Here's how the part is built. I have some questions about the finished solid (model axes, mm). Face numbers are marked on the shaded views. A direction names the side the tool comes from. Round coordinates to 2 decimals unless told otherwise and drop trailing zeros. Order: outer loops, then holes, each group sorted by start corner. A loop starts at its lowest first (then second) coordinate and runs counter-clockwise, first axis right, second up. Notation, with made-up numbers: (-3, 23.25) -> (56, 23.25) arc R8 cw to (56, 29.25) -> close; hole circle Ø2 at (70, -23). An arc over 180 degrees is marked (long way). Answer in a Markdown table with one row per item.
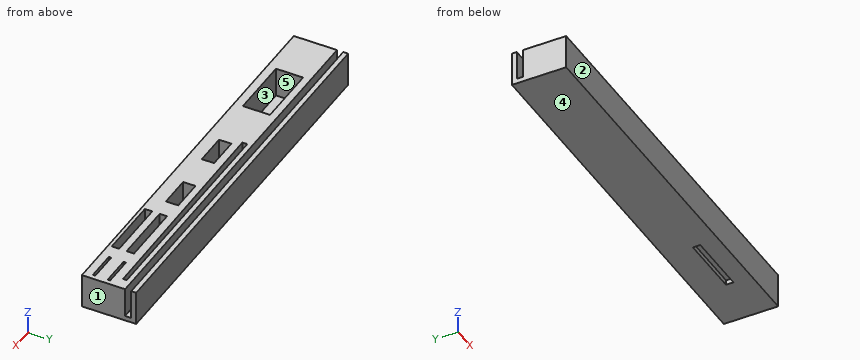
```python
from build123d import *

# Parameters (mm, degrees)
F0_W     = 160
F0_H     = 17.5
F0_W_2   = 25
F0_H_2   = 11
F0_W_3   = 13
F0_H_3   = 5
F0_H_4   = 3
F0_W_4   = 12
F0_H_5   = 1
F0_H_6   = 2.5
F0_H_7   = 2
F1_DEPTH = 2
F2_DEPTH = 12
F3_DEPTH = 2
F4_DEPTH = 2


# Not quite as in the source:
# - a feature names something its author has since deleted; it is built from what else it names


with BuildPart() as f1:
    # F0 (on Top) → F1 (new body)
    with BuildSketch(Plane.XY):
        with Locations((-35.2099549949, 29.3164705649)):
            Rectangle(F0_W, F0_H)
        with Locations((-82.7099549949, 29.5664705649)):
            Rectangle(F0_W_2, F0_H_2, mode=Mode.SUBTRACT)
        with Locations((-42.2099549949, 28.443671599)):
            Rectangle(F0_W_3, F0_H_3, mode=Mode.SUBTRACT)
        with Locations((12.2900450051, 23.443671599)):
            Rectangle(F0_W_2, F0_H_4, mode=Mode.SUBTRACT)
        with Locations((36.7900450051, 24.443671599)):
            Rectangle(F0_W_4, F0_H_5, mode=Mode.SUBTRACT)
        with Locations((-14.2099549949, 28.943671599)):
            Rectangle(F0_W_3, F0_H_3, mode=Mode.SUBTRACT)
        with Locations((12.2900450051, 29.443671599)):
            Rectangle(F0_W_2, F0_H_4, mode=Mode.SUBTRACT)
        with Locations((36.7900450051, 30.443671599)):
            Rectangle(F0_W_4, F0_H_5, mode=Mode.SUBTRACT)
        Polygon((-51.2099549949, 36.0664705649), (39.7900450051, 36.0664705649), (39.7900450051, 34.5664705649), (-51.2099549949, 34.0664705649), align=None, mode=Mode.SUBTRACT)
        with Locations((-35.2099549949, 39.3164705649)):
            Rectangle(F0_W, F0_H_6)
        with Locations((-35.2099549949, 41.5664705649)):
            Rectangle(F0_W, F0_H_7)
        with Locations((-82.7099549949, 29.5664705649)):
            Rectangle(F0_W_2, F0_H_2)
        Polygon((39.7900450051, 34.5664705649), (39.7900450051, 36.0664705649), (-51.2099549949, 36.0664705649), (-51.2099549949, 34.0664705649), align=None)
        with Locations((12.2900450051, 23.443671599)):
            Rectangle(F0_W_2, F0_H_4)
        with Locations((-42.2099549949, 28.443671599)):
            Rectangle(F0_W_3, F0_H_3)
        with Locations((-14.2099549949, 28.943671599)):
            Rectangle(F0_W_3, F0_H_3)
        with Locations((36.7900450051, 24.443671599)):
            Rectangle(F0_W_4, F0_H_5)
        with Locations((36.7900450051, 30.443671599)):
            Rectangle(F0_W_4, F0_H_5)
    extrude(amount=-F1_DEPTH)

    # F0 (on Top) → F2 (join)
    with BuildSketch(Plane.XY):
        with Locations((-35.2099549949, 29.3164705649)):
            Rectangle(F0_W, F0_H)
        with Locations((-82.7099549949, 29.5664705649)):
            Rectangle(F0_W_2, F0_H_2, mode=Mode.SUBTRACT)
        with Locations((-42.2099549949, 28.443671599)):
            Rectangle(F0_W_3, F0_H_3, mode=Mode.SUBTRACT)
        with Locations((12.2900450051, 23.443671599)):
            Rectangle(F0_W_2, F0_H_4, mode=Mode.SUBTRACT)
        with Locations((36.7900450051, 24.443671599)):
            Rectangle(F0_W_4, F0_H_5, mode=Mode.SUBTRACT)
        with Locations((-14.2099549949, 28.943671599)):
            Rectangle(F0_W_3, F0_H_3, mode=Mode.SUBTRACT)
        with Locations((12.2900450051, 29.443671599)):
            Rectangle(F0_W_2, F0_H_4, mode=Mode.SUBTRACT)
        with Locations((36.7900450051, 30.443671599)):
            Rectangle(F0_W_4, F0_H_5, mode=Mode.SUBTRACT)
        Polygon((-51.2099549949, 36.0664705649), (39.7900450051, 36.0664705649), (39.7900450051, 34.5664705649), (-51.2099549949, 34.0664705649), align=None, mode=Mode.SUBTRACT)
        with Locations((-35.2099549949, 41.5664705649)):
            Rectangle(F0_W, F0_H_7)
    extrude(amount=F2_DEPTH)

    # F0 (on Top) → F3 (join)
    with BuildSketch(Plane.XY):
        with Locations((36.7900450051, 30.443671599)):
            Rectangle(F0_W_4, F0_H_5)
        with Locations((36.7900450051, 24.443671599)):
            Rectangle(F0_W_4, F0_H_5)
    extrude(amount=F3_DEPTH)

    # F0 (on Top) → F4 (join)
    with BuildSketch(Plane.XY):
        with Locations((12.2900450051, 29.443671599)):
            Rectangle(F0_W_2, F0_H_4)
    extrude(amount=F4_DEPTH)


solid = f1.part
```
1. Suppose I cut it at B-B on x = -83. Write out the boundary of the cut face in (y, z).
Numbers:
| item | result |
|---|---|
| outline | (20.57, -2) -> (42.57, -2) -> (42.57, 12) -> (40.57, 12) -> (40.57, 0) -> (38.07, 0) -> (38.07, 12) -> (35.07, 12) -> (35.07, 0) -> (24.07, 0) -> (24.07, 12) -> (20.57, 12) -> close |
2. Suppose I cut it at D-D on x = -23.5. Write out the boundary of the cut face in (y, z), then the cut area to 3 significant figures.
Numbers:
| item | result |
|---|---|
| outline | (20.57, -2) -> (42.57, -2) -> (42.57, 12) -> (40.57, 12) -> (40.57, 0) -> (38.07, 0) -> (38.07, 12) -> (36.07, 12) -> (36.07, 0) -> (34.22, 0) -> (34.22, 12) -> (20.57, 12) -> close |
| area | 256 mm2 |
3. For the marked faces 4 and 5, which set-ups out of +Z, -Z, +X, -X, +Y, -Y let a thin tool reach every point of the face, with its end or its side?
Numbers:
| item | result |
|---|---|
| face 4 | -Z, +X, -X, +Y, -Y |
| face 5 | +Z |
4. We'd pull the mould along X, two halves only. Please class the marked faces 1, 2 and 3: released by +X, released by -X, zero draft, split by the parting line, or undercut.
Numbers:
| item | result |
|---|---|
| face 1 | released by +X |
| face 2 | zero draft |
| face 3 | undercut |
5. Please list where these lines run through material, in increasing order: line 1 along Y through (x, z) = (-46.5, 0.5); line 2 along X through (y, z) = (33.75, 3.75); line 3 along Y through (x, z) = (-23.5, 6.25).
Numbers:
| item | result |
|---|---|
| line 1 | y = 20.57 to 25.94, 30.94 to 34.09, 36.07 to 38.07, 40.57 to 42.57 |
| line 2 | x = -115.21 to -95.21, -70.21 to 44.79 |
| line 3 | y = 20.57 to 34.22, 36.07 to 38.07, 40.57 to 42.57 |
6. Suppose I cut it at C-C on x = 9.5. Write out the boundary of the cut face in (y, z), then the cut area to 3 significant figures.
Numbers:
| item | result |
|---|---|
| outline | (20.57, -2) -> (27.94, -2) -> (27.94, 0) -> (30.94, 0) -> (30.94, -2) -> (42.57, -2) -> (42.57, 12) -> (40.57, 12) -> (40.57, 0) -> (38.07, 0) -> (38.07, 12) -> (36.07, 12) -> (36.07, 0) -> (34.4, 0) -> (34.4, 12) -> (30.94, 12) -> (30.94, 2) -> (27.94, 2) -> (27.94, 12) -> (24.94, 12) -> (24.94, 0) -> (21.94, 0) -> (21.94, 12) -> (20.57, 12) -> close |
| area | 186 mm2 |
7. Suppose I cut it at A-A on z = 5.75. State how many separate pieces and enclosed holes the cut face has, then the cut area to 3 significant figures.
Numbers:
| item | result |
|---|---|
| separate pieces | 2 |
| enclosed holes | 8 |
| area | 2,380 mm2 |
